from build123d import *

# Parameters (mm, degrees)
F1_W     = 3.683
F1_H     = 3.683
F1_R     = 1.5875
F4_DEPTH = 3.683
F5_R     = 1.84149


# Not quite as in the source:
# - a fillet or chamfer is up to 0.001 mm smaller than in the source, because OpenCascade refuses the exact size


with BuildPart() as f2:
    # F2: sweep along a path in F0
    with BuildLine(Plane.XY) as f2_path:
        Line((0, 0), (0, 3.175))
        ThreePointArc((0, 3.175), (-1.7024337798, 7.2850387202), (-5.8124725, 8.9874725))
        Line((-5.8124725, 8.9874725), (-8.9874725, 8.9874725))
    # F1 (on Front) → F2 (sweep)
    with BuildSketch(Plane.XZ):
        Rectangle(F1_W, F1_H)
        Circle(F1_R, mode=Mode.SUBTRACT)
    sweep(path=f2_path.line)

    # F3 (on face) → F4 (cut, through all)
    with BuildSketch(Plane.XZ.offset(-7.1459725)):
        with BuildLine():
            Line((-8.9874725, 0), (-8.9874725, -0.933255592))
            ThreePointArc((-8.9874725, -0.933255592), (-8.7334725, 0), (-8.9874725, 0.933255592))
            Line((-8.9874725, 0.933255592), (-8.9874725, 0))
        make_face()
    extrude(amount=-F4_DEPTH, mode=Mode.SUBTRACT)

    # F5 (radius 1.8415 in the source; OpenCascade refuses exactly that, so slightly less here)
    f5_edges = [f2.edges().sort_by_distance(p)[0] for p in [
        (-3.004571, 5.982902, 1.8415),
        (-3.004571, 5.982902, -1.8415),
        (-0.400297, 8.587176, 1.8415),
        (-0.400297, 8.587176, -1.8415),
    ]]
    fillet(f5_edges, radius=F5_R)


solid = f2.part
Design review of the part built by this model. Coordinates are the model's own, in mm. A direction names the side the tool comes from. Round coordinates to 2 decimals unless told otherwise and drop trailing zeros. Write each loop counter-clockwise with the first axis right and the second up, starting at its lowest first coordinate (ties: lowest second). Pieces come first, ordered by that corner, then holes. Notation, with made-up numbers: (2, 16.25) - (17, 16.25) arc R26 cw to (17, 45.25) - close; hole circle Ø10 at (-3, -18). An arc over 180 degrees is marked (long way). Use a Markdown table: item, result. Add a question column.
1. Clearance check with flat-ended pins moving along their axes: pin 1 (1 mm diameter, centred on y = 6, z = -1, fed in from -X); pin 2 (1 mm diameter, centred on x = -2.5, z = 1.5, fed in from +Y); pin 3 (5 mm diameter, centred on x = -7, y = 3, fed in from +Z). State where each tip first meets the part, or that it passes through.
2. For faces 4 (the face through (-0.34, 1.61, 1.55)), 5 (the face through (-1.288, 1.61, 1.316)), 6 (the face through (-1.288, 1.61, -1.316)), list the 3-axis set-ups (+Z, -Z, +X, -X, +Y, -Y) from which the entire face can be reached by the end or side of a thin tool; tool diameter is ignored.
3. Wall thickness on probe 1 along X at (y, z) = (1.75, 0); probe 2 along X at (y, z) = (1.5, 0.55): over which ranges is each line inside the solid? List them lowest first.
4. We need section B-B (z = 0.25). State the section outline as (x, y) points (3 decimals), then the cut area to 3 significant figures.
5. We need section C-C (z = 1.25). State the section outline as (x, y) points (3 decimals), then the cut area to 3 significant figures.
6. Mouldability with a two-part tool opening along Z and no side actions: class faces 1 (the face through (-7.422, 10.275, 1.316)), 2 (the face through (-7.42, 8.64, 1.55)), 3 (the face through (-7.422, 7.7, -1.316)) as +Z half, -Z half, draft (parallel to the pull), parting line (faces both ways), or undercut.
Output:
| question | item | result |
|---|---|---|
| 1 | pin 1 | stops at x = -3.27 |
| 1 | pin 2 | stops at y = 9.82 |
| 1 | pin 3 | passes through |
| 2 | face 4 | -Y |
| 2 | face 5 | +Z, -X, -Y |
| 2 | face 6 | -Z, -X, -Y |
| 3 | probe 1 | x = -1.84 to -1.59, 1.59 to 1.84 |
| 3 | probe 2 | x = -1.76 to -1.49, 1.49 to 1.76 |
| 4 | outline | (-8.751, 7.163) - (-5.812, 7.163) arc R3.988 cw to (-1.824, 3.175) - (-1.824, 0) - (-1.568, 0) - (-1.568, 3.175) arc R4.245 ccw to (-5.812, 7.42) - (-8.751, 7.42) - close; (-8.751, 10.555) - (-5.812, 10.555) arc R7.38 cw to (1.568, 3.175) - (1.568, 0) - (1.824, 0) - (1.824, 3.175) arc R7.637 ccw to (-5.812, 10.812) - (-8.751, 10.812) - close |
| 4 | area | 7.83 mm2 |
| 5 | outline | (-8.987, 7.635) - (-5.812, 7.635) arc R4.46 cw to (-1.352, 3.175) - (-1.352, 0) - (-0.979, 0) - (-0.979, 3.175) arc R4.834 ccw to (-5.812, 8.009) - (-8.987, 8.009) - close; (-8.987, 9.966) - (-5.812, 9.966) arc R6.791 cw to (0.979, 3.175) - (0.979, 0) - (1.352, 0) - (1.352, 3.175) arc R7.165 ccw to (-5.812, 10.34) - (-8.987, 10.34) - close |
| 5 | area | 11.6 mm2 |
| 6 | face 1 | +Z half |
| 6 | face 2 | undercut |
| 6 | face 3 | -Z half |
